Geometry: see drawing. Coordinates: mm, zero at the bounding-box minimum. Round coordinates to 2 decimals unless told otherwise and drop trailing zeros. Loops run counter-clockwise (first coordinate to the right, second up) from the corner with the lowest first, then second, coordinate; pieces in that order, holes last.
(1) Section A-A, the plane x = 12.15. Return the cut outline in (y, z), plus the area to 3 significant figures.
(2) Mould query, pull axis X, two halves, no side actions, for the marked faces 1, 2 and 3. Classes: pulls with the +X half, pulls with the -X half, needs draft (parallel to the pull), parting line crosses it, or undercut.
(3) Section C-C, the plane y = 28.5. Return the cut outline in (x, z).
(4) First-contact query: pin 1 Ø1.5 at (x, y) = (13.5, 10) entering from -Z; pin 2 Ø2.5 at (x, z) = (12.15, 20.65) entering from +Y; pin 3 Ø4 at (x, y) = (6, 15) entering from -Z. Flat tips, straight axial feed; report the tip coordinate or a pass-through.
(5) Section B-B, the plane z = 12.15. Return the cut outline in (x, y).
(6) Material intervals for probe 1 along Z at (x, y) = (12.25, 4); probe 2 along X at (y, z) = (9.5, 12.25); probe 3 along Y at (x, z) = (21, 12.25), sorted ascending.
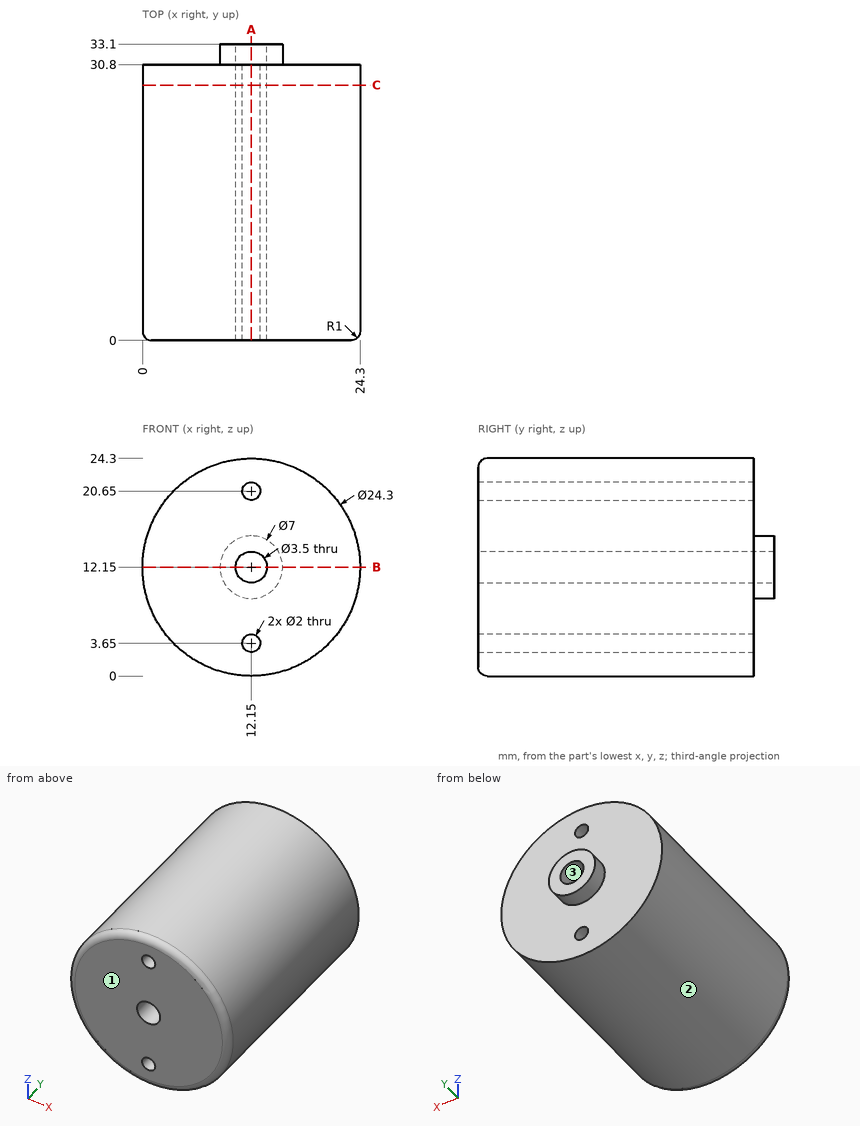
Output values:
1. outline: (0, 1) arc R1 ccw to (1, 0) - (30.8, 0) - (30.8, 2.65) - (0, 2.65) - close; (0, 4.65) - (30.8, 4.65) - (30.8, 8.65) - (33.1, 8.65) - (33.1, 10.4) - (0, 10.4) - close; (0, 13.9) - (33.1, 13.9) - (33.1, 15.65) - (30.8, 15.65) - (30.8, 19.65) - (0, 19.65) - close; (0, 21.65) - (30.8, 21.65) - (30.8, 24.3) - (1, 24.3) arc R1 ccw to (0, 23.3) - close
1. area: 525 mm2
2. face 1: needs draft
2. face 2: parting line crosses it
2. face 3: undercut
3. outline: circle Ø24.3 at (12.15, 12.15); hole circle Ø3.5 at (12.15, 12.15); hole circle Ø2 at (12.15, 3.65); hole circle Ø2 at (12.15, 20.65)
4. pin 1: stops at z = 0.01
4. pin 2: stops at y = 30.8
4. pin 3: stops at z = 0.73
5. outline: (0, 1) arc R1 ccw to (1, 0) - (10.4, 0) - (10.4, 33.1) - (8.65, 33.1) - (8.65, 30.8) - (0, 30.8) - close; (13.9, 0) - (23.3, 0) arc R1 ccw to (24.3, 1) - (24.3, 30.8) - (15.65, 30.8) - (15.65, 33.1) - (13.9, 33.1) - close
6. probe 1: z = 0 to 2.66, 4.64 to 10.4, 13.9 to 19.66, 21.64 to 24.3
6. probe 2: x = 0 to 10.4, 13.9 to 24.3
6. probe 3: y = 0 to 30.8
